CAD build for the part. Positions are in the model's coordinates, mm. A direction names the side the tool comes from. Round coordinates to 2 decimals unless told otherwise and drop trailing zeros. Loops run counter-clockwise (first coordinate to the right, second up) from the corner with the lowest first, then second, coordinate; pieces in that order, holes last.
```python
from build123d import *

# Parameters (mm, degrees)
SKETCH1_W                           = 80
SKETCH1_H                           = 80
BOSS_EXTRUDE1_DEPTH                 = 150
SKETCH2_W                           = 71.7
SKETCH2_H                           = 71.7
CUT_EXTRUDE1_71_7SQUARE_DEPTH       = 10
SKETCH4_W                           = 78
SKETCH4_H                           = 78
CUT_EXTRUDE2_COMPARTMENT1_6CM_DEPTH = 60
SKETCH5_W                           = 78
SKETCH5_H                           = 78
CUT_EXTRUDE3_DEPTH                  = 60
SKETCH6_W                           = 71
SKETCH6_H                           = 71
CUT_EXTRUDE4_DEPTH                  = 60
CUT_EXTRUDE4_TAPER                  = 2
CHAMFER1_SIZE                       = 6


with BuildPart() as part:
    # Sketch1 → Boss-Extrude1 (new body)
    with BuildSketch(Plane(origin=(0, 0, 0), x_dir=(0, 1, 0), z_dir=(0, 0, 1))):
        Rectangle(SKETCH1_W, SKETCH1_H)
    extrude(amount=BOSS_EXTRUDE1_DEPTH)

    # Sketch2 → Cut-Extrude1-71.7square (cut)
    with BuildSketch(Plane.XY.offset(150)):
        Rectangle(SKETCH2_W, SKETCH2_H)
    extrude(amount=-CUT_EXTRUDE1_71_7SQUARE_DEPTH, mode=Mode.SUBTRACT)

    # Sketch4 → Cut-Extrude2-compartment1-6cm (cut)
    with BuildSketch(Plane.XY.offset(137)):
        with Locations((1, -1)):
            Rectangle(SKETCH4_W, SKETCH4_H)
    extrude(amount=-CUT_EXTRUDE2_COMPARTMENT1_6CM_DEPTH, mode=Mode.SUBTRACT)

    # Sketch5 → Cut-Extrude3 (cut)
    with BuildSketch(Plane.XY.offset(73)):
        with Locations((1, -1)):
            Rectangle(SKETCH5_W, SKETCH5_H)
    extrude(amount=-CUT_EXTRUDE3_DEPTH, mode=Mode.SUBTRACT)

    # Sketch6 → Cut-Extrude4 (cut)
    with BuildSketch(Plane(origin=(0, 0, 10), x_dir=(1, 0, 0), z_dir=(0, 0, -1))):
        Rectangle(SKETCH6_W, SKETCH6_H)
    extrude(amount=CUT_EXTRUDE4_DEPTH, taper=CUT_EXTRUDE4_TAPER, mode=Mode.SUBTRACT)

    # Chamfer1
    chamfer1_edges = [part.edges().sort_by_distance(p)[0] for p in [
        (40, -40, 75),
        (40, -40, 6.5),
        (40, -40, 143.5),
    ]]
    chamfer(chamfer1_edges, length=CHAMFER1_SIZE)


solid = part.part
```
Item 1: Cut at A-A, the plane z = 130.5. Give the cut face in (x, y), plus the area to 3 significant figures.
Answers follow:
outline: (-40, -40) - (-38, -40) - (-38, 38) - (40, 38) - (40, 40) - (-40, 40) - close
area: 316 mm2
Item 2: Two-plate mould, pull along X, no slides. Class faces 1 (the flat face through (-39, 0, 150)), 2 (the flat face through (-1, 35.85, 145)), 3 (the flat face through (-38, -2, 43)): released by +X, released by -X, zero draft, split by the parting line, or undercut.
Answers follow:
face 1: zero draft
face 2: undercut
face 3: released by +X
Item 3: Flat gauge pins, fed straight in: P1, Ø1.5, axis at x = 8, y = -27, coming from the +Z side; P2, Ø1, axis at x = -6, z = 28.5, coming from the -Y side; P3, Ø2, axis at x = 26, y = 31.5, coming from the -Z side. Where does each tip first touch, or does it go through?
Answers follow:
P1: stops at z = 140
P2: stops at y = 38
P3: stops at z = 10
Item 4: Probe line 1 (Z direction, x = 29.5, y = -16); line 2 (Z direction, x = 18, y = 36.5); line 3 (Y direction, x = 6, z = 116). List the from-to ranges inside material, lowest first.
Answers follow:
line 1: z = 10 to 13, 73 to 77, 137 to 140
line 2: z = 0 to 13, 73 to 77, 137 to 150
line 3: y = 38 to 40
Item 5: 3-axis set-ups, long thin cutter, end or side, ignore diameter. For faces 4 (the flat face through (-8, -40, 75)), 5 (the flat face through (0, 38, 43)), 6 (the flat face through (35.85, -1, 145)): which of +Z, -Z, +X, -X, +Y, -Y reach the whole face in a straight line?
Answers follow:
face 4: +Z, -Z, +X, -X, -Y
face 5: +X, -Y
face 6: +Z
